Autodesk Inventor part; units mm, degrees
ref_plane "YZ Plane" through (0, 0, 0) normal (1, 0, 0) x (0, 1, 0)
ref_plane "XZ Plane" through (0, 0, 0) normal (0, 1, 0) x (-1, 0, 0)
ref_plane "XY Plane" through (0, 0, 0) normal (0, 0, 1) x (1, 0, 0)
sketch "Sketch1" plane through (0, 0, 0) normal (0, 1, 0) x (-1, 0, 0)
  line L0 (-7.5, 9) -> (7.5, 9)
  line L1 (7.5, 9) -> (7.5, -9)
  line L2 (7.5, -9) -> (-7.5, -9)
  line L3 (-7.5, -9) -> (-7.5, 9)
  line L4 (-7.5, 9) -> (7.5, -9) construction
  line L5 (7.5, 9) -> (-7.5, -9) construction
  point P0 (0, 0)
  dimension "d0" = 18
  dimension "d1" = 15
extrude "Extrusion1" add sketch "Sketch1" along normal blind 25.4
sketch "Sketch2" plane through (0, 25.4, 0) normal (0, 1, 0) x (1, 0, 0)
  line L0 (12.4357, -5) -> (-12.4357, -5)
  line L1 (-12.4357, -5) -> (-12.4357, 5)
  line L2 (-12.4357, 5) -> (12.4357, 5)
  line L3 (12.4357, 5) -> (12.4357, -5)
  line L4 (12.4357, -5) -> (-12.4357, 5) construction
  line L5 (-12.4357, -5) -> (12.4357, 5) construction
  line L6 (7.5, 9) -> (-7.5, 9)
  point P0 (0, 0)
  dimension "d5" = 10
extrude "Extrusion2" cut sketch "Sketch2" against normal blind 19.05
sketch "Sketch3" plane through (7.5, 0, -9) normal (0, 0, -1) x (-1, 0, 0)
  line L0 (0, 25.4) -> (15, 25.4)
  line L1 (7.5, 25.4) -> (7.5, 0)
  circle A0 centre (7.5, 19.9547) radius 1.5
  dimension "d8" = 3
extrude "Extrusion3" cut sketch "Sketch3" against normal through all
fillet "Fillet1" radius 3.175 4 edges at (-7.5, 25.4, -7) (7.5, 25.4, -7) (-7.5, 25.4, 7) (7.5, 25.4, 7)
sketch "Sketch4" plane through (0, 0, 0) normal (0, -1, 0) x (1, 0, 0)
  circle A0 centre (0, 0) radius 2.75
  dimension "d12" = 5.5
extrude "Extrusion4" cut sketch "Sketch4" against normal blind 19.05
sketch "Sketch5" plane through (0, 6.35, 0) normal (0, 1, 0) x (1, 0, 0)
  line L0 (-4.6188, 0) -> (-2.3094, 4)
  line L1 (-2.3094, 4) -> (2.3094, 4)
  line L2 (2.3094, 4) -> (4.6188, 0)
  line L3 (4.6188, 0) -> (2.3094, -4)
  line L4 (2.3094, -4) -> (-2.3094, -4)
  line L5 (-2.3094, -4) -> (-4.6188, 0)
  point P0 (0, 0)
  point P1 (0, 0)
  dimension "d15" = 8
extrude "Extrusion5" cut sketch "Sketch5" against normal blind 2.54
sketch "Sketch6" plane through (-7.5, 0, 9) normal (0, 0, 1) x (1, 0, 0)
  circle A0 centre (7.5, 19.9547) radius 1.5
  circle A1 centre (7.5, 19.9547) radius 3
  point P0 (7.5, 0)
  dimension "d18" = 6
extrude "Extrusion6" cut sketch "Sketch6" against normal blind 2.5
sketch "Sketch7" plane through (7.5, 0, -9) normal (0, 0, -1) x (-1, 0, 0)
  circle A0 centre (7.5, 19.9547) radius 1.5
  line L0 (10.6129, 19.0812) -> (8.3, 16.822)
  line L1 (8.3, 16.822) -> (5.1871, 17.6955)
  line L2 (5.1871, 17.6955) -> (4.3871, 20.8282)
  line L3 (4.3871, 20.8282) -> (6.7, 23.0873)
  line L4 (6.7, 23.0873) -> (9.8129, 22.2138)
  line L5 (9.8129, 22.2138) -> (10.6129, 19.0812)
  point P0 (7.5, 0)
  dimension "d21" = 5.6
extrude "Extrusion7" cut sketch "Sketch7" against normal blind 2.5
sketch "Sketch8" plane through (7.5, 0, -9) normal (0, 0, -1) x (-1, 0, 0)
  line L0 (9.8129, 22.2138) -> (10.6129, 19.0812)
  line L1 (10.6129, 19.0812) -> (8.3, 16.822)
  line L2 (8.3, 16.822) -> (5.1871, 17.6955)
  line L3 (5.1871, 17.6955) -> (4.3871, 20.8282)
  line L4 (4.3871, 20.8282) -> (6.7, 23.0873)
  line L5 (6.7, 23.0873) -> (9.8129, 22.2138)
  arc A0 (3.175, 25.4) -> (0, 22.225) centre (3.175, 22.225) ccw
  line L6 (0, 0) -> (0, 22.225)
  line L7 (15, 0) -> (0, 0)
  line L8 (15, 0) -> (15, 22.225)
  arc A1 (15, 22.225) -> (11.825, 25.4) centre (11.825, 22.225) ccw
  line L9 (3.175, 25.4) -> (11.825, 25.4)
  point P0 (7.5, 0)
extrude "Extrusion8" add sketch "Sketch8" along normal blind 1
sketch "Sketch9" plane through (-7.5, 0, 9) normal (0, 0, 1) x (1, 0, 0)
  circle A0 centre (7.5, 19.9547) radius 3
  arc A1 (15, 22.225) -> (11.825, 25.4) centre (11.825, 22.225) ccw
  line L0 (3.175, 25.4) -> (11.825, 25.4)
  arc A2 (3.175, 25.4) -> (0, 22.225) centre (3.175, 22.225) ccw
  line L1 (0, 0) -> (0, 22.225)
  line L2 (15, 0) -> (0, 0)
  line L3 (15, 0) -> (15, 22.225)
  point P0 (7.5, 0)
extrude "Extrusion9" add sketch "Sketch9" along normal blind 1
properties part number "xTension"
Here's how the part is built. I have some questions about the finished solid (model axes, mm). A direction names the side the tool comes from. Round coordinates to 2 decimals unless told otherwise and drop trailing zeros. Loops run counter-clockwise (first coordinate to the right, second up) from the corner with the lowest first, then second, coordinate; pieces in that order, holes last.
1. We'd pull the mould along Y, two halves only. Please class faces 1 (the face through (0, 25.4, -7)), 2 (the face through (1.973, 21.942, -8.226)), 3 (the face through (0, 16, 5)): +Y half, -Y half, draft (parallel to the pull), parting line (faces both ways), or undercut.
Answer list:
face 1: +Y half
face 2: undercut
face 3: draft
2. If we section it at D-D on z = 7.25: Write out the boundary of the cut face in (x, y) (3 decimals).
Answer list:
outline: (-7.5, 0) - (7.5, 0) - (7.5, 22.225) arc R3.175 ccw to (4.325, 25.4) - (-4.325, 25.4) arc R3.175 ccw to (-7.5, 22.225) - close; hole circle Ø6 at (0, 19.955)
3. If we section it at A-A on y = 5.75: Write out the boundary of the cut face in (x, z).
Answer list:
outline: (-7.5, -10) - (7.5, -10) - (7.5, 10) - (-7.5, 10) - close; hole (-4.62, 0) - (-2.31, -4) - (2.31, -4) - (4.62, 0) - (2.31, 4) - (-2.31, 4) - close
4. Which directions (+Z, -Z, +X, -X, +Y, -Y) give clear straight access to the entire face, cutting with the end or side of a thin tool? Please do faces 4 (the face through (0.73, 17.25, -8.23)), 5 (the face through (0, 16, -5)), 6 (the face through (3.48, 5.1, 1.97)).
Answer list:
face 4: -Z
face 5: +X, -X, +Y
face 6: +Y
5. If we section it at B-B on x = 0: Count the separate pieces of the cut face and the enclosed holes in it, plus the area to 3 significant figures.
Answer list:
separate pieces: 4
enclosed holes: 0
area: 226 mm2
6. If I drill on line 1 along Z through (x, y) = (6.5, 22.75); line 2 along Y through (x, z) = (0, 5.8); line 3 along Y through (x, z) = (0, 9.15), over which ranges is the centre line in solid material (lowest first)?
Answer list:
line 1: z = -10 to -5, 5 to 10
line 2: y = 0 to 18.45, 21.45 to 25.4
line 3: y = 0 to 16.95, 22.95 to 25.4
7. For P1, Ø3, axis at x = 1, y = 20, coming from the +Z side; P2, Ø2.5, axis at x = 0, y = 19.95, coming from the +Z side; P3, Ø1.9, axis at x = 0.5, y = 20.5, coming from the -Z side; P4, Ø5, axis at x = 0.5, z = 1, coming from the +Y side, each with a flat end and sliding along its axis, tell me the tip position at first contact or that it passes through.
Answer list:
P1: stops at z = 6.5
P2: passes through
P3: stops at z = -6.5
P4: stops at y = 3.81
8. If we section it at C-C on y = 8.5: Write out the boundary of the cut face in (x, z), plus the area to 3 significant figures.
Answer list:
outline: (-7.5, -10) - (7.5, -10) - (7.5, -5) - (-7.5, -5) - close; (-7.5, 5) - (7.5, 5) - (7.5, 10) - (-7.5, 10) - close
area: 150 mm2
